Solid Edge part; units mm, degrees
sketch "Sketch1" plane through (0, 0, 15) normal (0, 0, 1) x (1, 0, 0)
  line L0 (-92, 52.0628) -> (-92, -46)
  arc A0 (-92, -46) -> (-87, -51) centre (-87, -46) ccw
  line L1 (-87, -51) -> (87, -51)
  arc A1 (87, -51) -> (92, -46) centre (87, -46) ccw
  line L2 (92, -46) -> (92, 52.0628)
  arc A2 (92, 52.0628) -> (89.4807, 56.404) centre (87, 52.0628) ccw
  line L3 (89.4807, 56.404) -> (33.7798, 88.2331)
  arc A3 (33.7798, 88.2331) -> (23.3609, 91) centre (23.3609, 70) ccw
  line L4 (23.3609, 91) -> (-23.3609, 91)
  arc A4 (-23.3609, 91) -> (-33.7798, 88.2331) centre (-23.3609, 70) ccw
  line L5 (-33.7798, 88.2331) -> (-89.4807, 56.404)
  arc A5 (-89.4807, 56.404) -> (-92, 52.0628) centre (-87, 52.0628) ccw
extrude "Protrusion1" add sketch "Sketch1" along normal blind 3
hole "Bohrung_1" at (-86, 51.4825, 18) direction (0, 0, -1) diameter 3.2 end through all countersink diameter 6.94 countersink angle 90
hole "Hole1" at (86, 51.4825, 18) direction (0, 0, -1) diameter 3.2 end through all countersink diameter 6.94 countersink angle 90
hole "Hole2" at (86, -45, 18) direction (0, 0, -1) diameter 3.2 end through all countersink diameter 6.94 countersink angle 90
hole "Hole3" at (-86, -45, 18) direction (0, 0, -1) diameter 3.2 end through all countersink diameter 6.94 countersink angle 90
sketch "Sketch2" plane through (0, 20, 18) normal (0, 0, 1) x (1, 0, 0)
  circle A0 centre (70, 25) radius 8
extrude "Cutout1" cut sketch "Sketch2" against normal through all
Work out the finished part from the listing and answer in its coordinate system (mm). Give positions to 0.01 mm unless a question says otherwise; leave off trailing zeros. Order: outer loops, then holes, each group sorted by start corner. A loop starts at its lowest first (then second) coordinate and runs counter-clockwise, first axis right, second up. Notation, with made-up numbers: (59, 69) - (65, 69) arc R34 cw to (65, 101) - close; hole circle Ø11 at (3, 8.5). An arc over 180 degrees is marked (long way). Answer as CSV lines item,"result". Start each with the question number.
Q1. Given pin 1 Ø4 at (x, y) = (86, 51.48) entering from +Z; pin 2 Ø3.5 at (x, y) = (-86, -45) entering from +Z; pin 3 Ø4 at (x, y) = (86, -45) entering from -Z; pin 4 Ø2.5 at (x, y) = (-86, 51.48) entering from -Z, each flat-ended and moving along its own axis, determine where each tip first touches the part or whether it passes through.
Q2. Find the intervals of material crossed by L1, parallel to Y at x = -86, z = 15.35; L2, parallel to X at y = 53.5, z = 17.15; L3, parallel to Y at x = -85, z = 16.5, in increasing order. Write a range as [from, to].
Q3. The part is cut by section A-A (x = 70). Write down the section's boundary in (y, z), then the cut area to 3 significant figures.
Q4. The part is cut by section C-C (x = -65). Write down the section's boundary in (y, z), then the cut area to 3 significant figures.
Q5. The part is cut by section B-B (z = 17.2). Write down the section's boundary in (x, y), then the cut area to 3 significant figures.
Q6. The mould has two halves that part along Y. Classify faces 1 (the face through (-1, 21, 15)), 2 (the face through (91, -49, 16)), 3 (the face through (86.52, -46.64, 16.25)): +Y half, -Y half, draft (parallel to the pull), parting line (faces both ways), or undercut.
Check result:
1,pin 1,"stops at z = 16.53"
1,pin 2,"stops at z = 16.28"
1,pin 3,"stops at z = 15"
1,pin 4,"passes through"
2,L1,"y = [-51, -46.6], [-43.4, 49.88], [53.08, 58.39]"
2,L2,"x = [-91.79, -87.67], [-84.33, 84.33], [87.67, 91.79]"
2,L3,"y = [-51, -46.7], [-43.3, 49.79], [53.18, 58.96]"
3,outline,"(-51, 15) - (37, 15) - (37, 18) - (-51, 18) - close; (53, 15) - (67.54, 15) - (67.54, 18) - (53, 18) - close"
3,area,"308 mm²"
4,outline,"(-51, 15) - (70.39, 15) - (70.39, 18) - (-51, 18) - close"
4,area,"364 mm²"
5,outline,"(-92, -46) arc R5 ccw to (-87, -51) - (87, -51) arc R5 ccw to (92, -46) - (92, 52.06) arc R5 ccw to (89.48, 56.4) - (33.78, 88.23) arc R21 ccw to (23.36, 91) - (-23.36, 91) arc R21 ccw to (-33.78, 88.23) - (-89.48, 56.4) arc R5 ccw to (-92, 52.06) - close; hole circle Ø5.34 at (-86, -45); hole circle Ø5.34 at (-86, 51.48); hole circle Ø16 at (70, 45); hole circle Ø5.34 at (86, -45); hole circle Ø5.34 at (86, 51.48)"
5,area,"23,500 mm²"
6,face 1,"draft"
6,face 2,"-Y half"
6,face 3,"undercut"
